Design review of the part built by this model. Coordinates are the model's own, in mm. A direction names the side the tool comes from. Round coordinates to 2 decimals unless told otherwise and drop trailing zeros. Loops run counter-clockwise (first coordinate to the right, second up) from the corner with the lowest first, then second, coordinate; pieces in that order, holes last. Notation, with made-up numbers: (78.5, -9) - (92.5, -9) arc R31 ccw to (92.5, 30) - close; hole circle Ø4 at (54.25, -19). An arc over 180 degrees is marked (long way). Use one line per item in the form item = value. Start each with the question number.
(1) We need section D-D, the plane x = 3.5. Write out the cut boundary in (y, z), then the cut area to 3 significant figures.
(2) The part is to be moulded in two halves that separate along Z. For faces 1 (the cylindrical face through (0.887, 7.91, -10.316)), 2 (the flat face through (0, 13.1, 1.2)), say which applies: released by +Z, released by -Z, zero draft, split by the parting line, or undercut.
(3) We need section C-C, the plane x = 8.25. Write out the cut boundary in (y, z), then the cut area to 3 significant figures.
(4) Machinability: for faces 3 (the cylindrical face through (6.313, -0.66, -14.985)), 4 (the cylindrical face through (10.93, -4.48, 14.21)), 5 (the flat face through (12.5, 16, 0)), which of the approach directions +Z, -Z, +X, -X, +Y, -Y give a long, thin tool a straight path to every point of the face, cutting with its end or side? Answer none if there is none.
(5) Wall thickness on probe 1 along Z at (x, y) = (6, 0); probe 2 along Z at (x, y) = (4.5, -3.5); probe 3 along Y at (x, z) = (10.8, 0): over which ranges is each line inside the solid? List them lowest first. Write a range as [from, to].
(6) We need section A-A, the plane z = 0. Write out the cut boundary in (x, y), then the cut area to 3 significant figures.
(7) For pin 1 (15 mm diameter, centred on y = 2.5, z = 0, fed in from +X); pin 2 (5 mm diameter, centred on x = 10.5, z = 8, fed in from -Y); pin 3 (1 mm diameter, centred on x = 10.5, z = -12.5, fed in from +Y); pin 4 (6 mm diameter, centred on x = 10, z = -17.5, fed in from +Y), all flat-tipped, find the tip position at first contact; note any pin that passes through.
from build123d import *

# Parameters (mm, degrees)
F2_SIZE2 = 1.3856406461
F2_SIZE  = 0.8


with BuildPart() as f1:
    # F0 (on Front) → F1 (revolve)
    with BuildSketch(Plane.XZ):
        with BuildLine():
            Line((6.3, 24), (6.2, 24))
            ThreePointArc((6.2, 24), (1.8159379566, 22.1840620434), (0, 17.8))
            Line((0, 17.8), (0, 13))
            Line((0, 13), (1.75, 13))
            Line((1.75, 13), (1.75, 15))
            Line((1.75, 15), (10.75, 15))
            Line((10.75, 15), (10.75, 14.9))
            Line((10.75, 14.9), (12.5, 14.9))
            Line((12.5, 14.9), (12.5, 17.8))
            ThreePointArc((12.5, 17.8), (10.6840620434, 22.1840620434), (6.3, 24))
        make_face()
    revolve(axis=Axis((16.1859672517, 0, 0), (1, 0, 0)))

    # F2
    f2_edges = [f1.edges().sort_by_distance(p)[0] for p in [
        (12.5, 0, -14.9),
    ]]
    f2_side = f1.faces().sort_by_distance((12.5, 0, -15.40346))[0]
    chamfer(f2_edges, length=F2_SIZE, length2=F2_SIZE2, reference=f2_side)


solid = f1.part
Data:
q1.outline = circle Ø46.76 at (0, 0); hole circle Ø30 at (0, 0)
q1.area = 1,010 mm^2
q2.face_1 = undercut
q2.face_2 = zero draft
q3.outline = circle Ø47.37 at (0, 0); hole circle Ø30 at (0, 0)
q3.area = 1,060 mm^2
q4.face_3 = none
q4.face_4 = +X
q4.face_5 = +Z, -Z, +X, +Y, -Y
q5.probe_1 = [-24, -15], [15, 24]
q5.probe_2 = [-23.5, -14.59], [14.59, 23.5]
q5.probe_3 = [-22.06, -14.9], [14.9, 22.06]
q6.outline = (0, -17.8) arc R6.2 ccw to (6.2, -24) - (6.3, -24) arc R6.2 ccw to (12.5, -17.8) - (12.5, -15.7) - (11.11, -14.9) - (10.75, -14.9) - (10.75, -15) - (1.75, -15) - (1.75, -13) - (0, -13) - close; (0, 13) - (1.75, 13) - (1.75, 15) - (10.75, 15) - (10.75, 14.9) - (11.11, 14.9) - (12.5, 15.7) - (12.5, 17.8) arc R6.2 ccw to (6.3, 24) - (6.2, 24) arc R6.2 ccw to (0, 17.8) - close
q6.area = 198 mm^2
q7.pin_1 = through
q7.pin_2 = -22.68
q7.pin_3 = 19.14
q7.pin_4 = 18.3
